Job drawing, mm, ordinate dimensions from the low corner. One solid piece. A direction names the side the tool comes from. Round coordinates to 2 decimals unless told otherwise and drop trailing zeros. Loops run counter-clockwise (first coordinate to the right, second up) from the corner with the lowest first, then second, coordinate; pieces in that order, holes last.
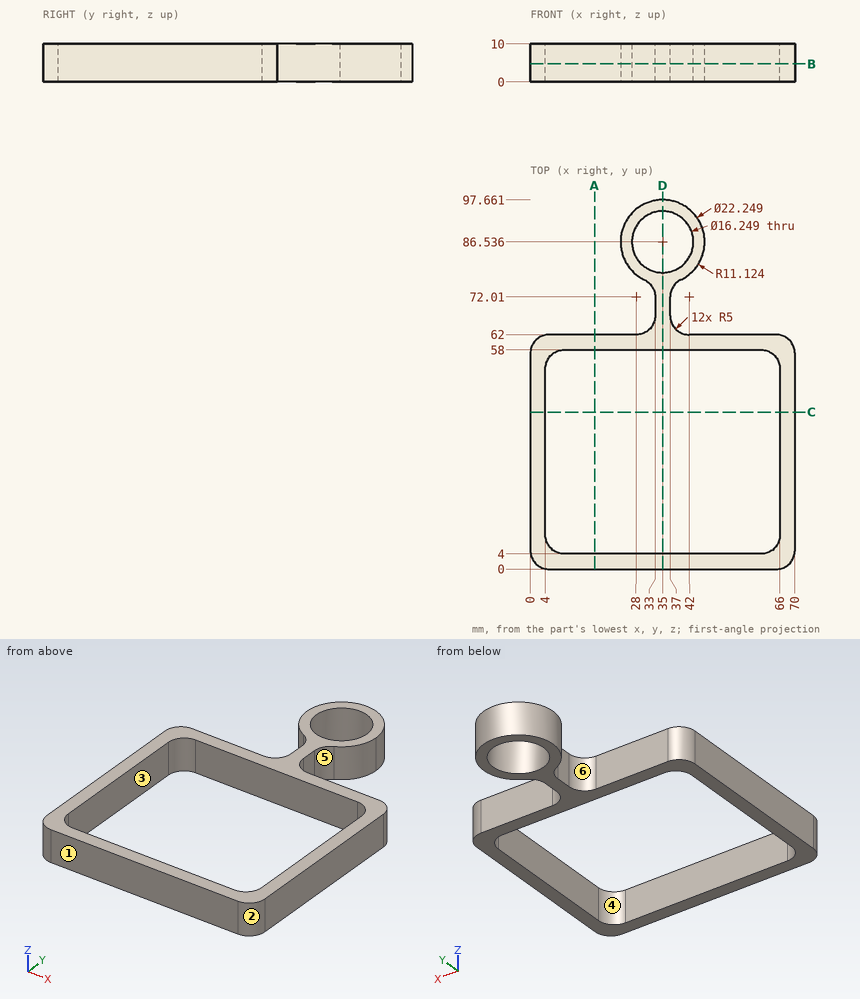
Item 1: 3-axis set-ups, long thin cutter, end or side, ignore diameter. For the marked faces 4, 5 and 6: which of +Z, -Z, +X, -X, +Y, -Y reach the whole face in a straight line?
Answers follow:
face 4: +Z, -Z
face 5: +Z, -Z, +X
face 6: +Z, -Z, -X
Item 2: Cut at D-D, the plane x = 35. Give the cut face in (y, z), plus the area to 3 significant figures.
Answers follow:
outline: (0, 0) - (4, 0) - (4, 10) - (0, 10) - close; (58, 0) - (78.41, 0) - (78.41, 10) - (58, 10) - close; (94.66, 0) - (97.66, 0) - (97.66, 10) - (94.66, 10) - close
area: 274 mm2
Item 3: Flat gauge pins, fed straight in: P1, Ø12, axis at x = 32, y = 68.5, coming from the +Z side; P2, Ø2.5, axis at y = 69, z = 2.5, coming from the +X side; P3, Ø2.5, axis at y = 70, z = 6.5, coming from the -X side; P4, Ø2, axis at x = 39.5, z = 2.5, coming from the +Y side (1 decimal). Where does each tip first touch, or does it go through?
Answers follow:
P1: stops at z = 10
P2: stops at x = 37
P3: stops at x = 33
P4: stops at y = 97.1
Item 4: Cut at C-C, the plane y = 41.5. Give the cut face in (x, z).
Answers follow:
outline: (0, 0) - (4, 0) - (4, 10) - (0, 10) - close; (66, 0) - (70, 0) - (70, 10) - (66, 10) - close
Item 5: Two-plate mould, pull along X, no slides. Class the marked faces 1, 2 and 3: released by +X, released by -X, zero draft, split by the parting line, or undercut.
Answers follow:
face 1: zero draft
face 2: released by +X
face 3: undercut
Item 6: Probe line 1 (Y direction, x = 35, z = 7); line 2 (X direction, y = 15, z = 4); line 3 (Y direction, x = 59.5, z = 3.5). List the from-to ranges inside material, lowest first.
Answers follow:
line 1: y = 0 to 4, 58 to 78.41, 94.66 to 97.66
line 2: x = 0 to 4, 66 to 70
line 3: y = 0 to 4, 58 to 62
Item 7: Cut at A-A, the plane x = 17. Give the cut face in (y, z).
Answers follow:
outline: (0, 0) - (4, 0) - (4, 10) - (0, 10) - close; (58, 0) - (62, 0) - (62, 10) - (58, 10) - close
Item 8: Cut at B-B, the plane z = 4.75. State how many separate pieces and enclosed holes the cut face has, plus the area to 3 significant figures.
Answers follow:
separate pieces: 1
enclosed holes: 2
area: 1,240 mm2
